Check sheet for the modelled part. Datum: model origin and axes. Units: mm. Give positions to 0.01 mm unless a question says otherwise; leave off trailing zeros. Loops run counter-clockwise (first coordinate to the right, second up) from the corner with the lowest first, then second, coordinate; pieces in that order, holes last. Notation, with made-up numbers: (70, 3.25) -> (128, 3.25) arc R20 ccw to (128, 12.25) -> close; hole circle Ø1 at (76, 86.5). An arc over 180 degrees is marked (long way). Answer as CSV lines item,"result". Start each with the question number.
(1) Gauge pin test, flat ends, axial feed: pin 1 Ø4 at (x, y) = (16, 0.58) entering from -Z; pin 2 Ø5 at (x, y) = (-24, -8) entering from -Z; pin 3 Ø6 at (x, y) = (8, -8) entering from -Z; pin 4 Ø7 at (x, y) = (0, 0.58) entering from -Z. Record the tip position at first contact, or that the pin passes through.
(2) Material ranges on line 1 (Y direction, x = -24, z = 3.15); line 2 (X direction, y = 8, z = 3.2); line 3 (Y direction, x = 9, z = 3.6), recorded low to high. Write a range as from..to.
(3) Section check B-B on x = 65. Enter the section's corners in (y, z), plus the area to 3 significant figures.
(4) Section check C-C on x = -16. Enter the section's corners in (y, z).
(5) Section check A-A on x = 24. Enter the section's corners in (y, z), plus the area to 3 significant figures.
from build123d import *

# Parameters (mm, degrees)
ESQUISSE1_W                                 = 150
ESQUISSE1_H                                 = 30
BOSS_EXTRU_1_DEPTH                          = 4
FRAISAGE_POUR_VIS_T_TE_FRAIS_E_M41_AT_COUNT = 2
FRAISAGE_POUR_VIS_T_TE_FRAIS_E_M41_AT_PITCH = 16
FRAISAGE_POUR_VIS_T_TE_FRAIS_E_M41_2_COUNT  = 2
FRAISAGE_POUR_VIS_T_TE_FRAIS_E_M41_2_PITCH  = 10.908274416
FRAISAGE_POUR_VIS_T_TE_FRAIS_E_M41_3_COUNT  = 2
FRAISAGE_POUR_VIS_T_TE_FRAIS_E_M41_3_PITCH  = 10.908274416
FRAISAGE_POUR_VIS_T_TE_FRAIS_E_M41_4_COUNT  = 2
FRAISAGE_POUR_VIS_T_TE_FRAIS_E_M41_4_PITCH  = 16
FRAISAGE_POUR_VIS_T_TE_FRAIS_E_M41_5_COUNT  = 2
FRAISAGE_POUR_VIS_T_TE_FRAIS_E_M41_5_PITCH  = 22.627416998
FRAISAGE_POUR_VIS_T_TE_FRAIS_E_M41_6_COUNT  = 2
FRAISAGE_POUR_VIS_T_TE_FRAIS_E_M41_6_PITCH  = 25.119523298
FRAISAGE_POUR_VIS_T_TE_FRAIS_E_M41_7_COUNT  = 2
FRAISAGE_POUR_VIS_T_TE_FRAIS_E_M41_7_PITCH  = 16
FRAISAGE_POUR_VIS_T_TE_FRAIS_E_M41_8_COUNT  = 2
FRAISAGE_POUR_VIS_T_TE_FRAIS_E_M41_8_PITCH  = 25.119523298
FRAISAGE_POUR_VIS_T_TE_FRAIS_E_M41_9_COUNT  = 2
FRAISAGE_POUR_VIS_T_TE_FRAIS_E_M41_9_PITCH  = 22.627416998
FRAISAGE_POUR_VIS_T_TE_FRAIS_E_M41_10_COUNT = 2
FRAISAGE_POUR_VIS_T_TE_FRAIS_E_M41_10_PITCH = 32
FRAISAGE_POUR_VIS_T_TE_FRAIS_E_M41_11_COUNT = 2
FRAISAGE_POUR_VIS_T_TE_FRAIS_E_M41_11_PITCH = 40.681573848
FRAISAGE_POUR_VIS_T_TE_FRAIS_E_M41_12_COUNT = 2
FRAISAGE_POUR_VIS_T_TE_FRAIS_E_M41_12_PITCH = 35.77708764
D_GAGEMENT_M61_D                            = 6.6
CONG_1_R                                    = 8
CHANFREIN1_SIZE                             = 0.5


with BuildPart() as part:
    # Esquisse1 → Boss.-Extru.1 (new body)
    with BuildSketch(Plane.XY):
        Rectangle(ESQUISSE1_W, ESQUISSE1_H)
    extrude(amount=BOSS_EXTRU_1_DEPTH)

    # Esquisse3 → Fraisage pour vis à tête fraisée M41 (revolve, cut)
    with BuildSketch(Plane(origin=(8, 8, 0), x_dir=(0, 1, 0), z_dir=(1, 0, 0))):
        Polygon((0, 0), (0, 4), (2.25, 4), (2.25, 2.45), (4.7, 0), align=None)
    fraisage_pour_vis_t_te_frais_e_m41 = revolve(axis=Axis((8, 8, -6.35), (0, 0, 1)), mode=Mode.SUBTRACT)

    # Fraisage pour vis à tête fraisée M41 at: Fraisage pour vis à tête fraisée M41 ×2
    with Locations(*[(0, -i * FRAISAGE_POUR_VIS_T_TE_FRAIS_E_M41_AT_PITCH, 0) for i in range(1, FRAISAGE_POUR_VIS_T_TE_FRAIS_E_M41_AT_COUNT)]):
        add(fraisage_pour_vis_t_te_frais_e_m41, mode=Mode.SUBTRACT)

    # Fraisage pour vis _ t_te frais_e M41 2: Fraisage pour vis à tête fraisée M41 ×2
    with Locations(*[Vector(0.733388224, -0.679810057, 0) * (i * FRAISAGE_POUR_VIS_T_TE_FRAIS_E_M41_2_PITCH) for i in range(1, FRAISAGE_POUR_VIS_T_TE_FRAIS_E_M41_2_COUNT)]):
        add(fraisage_pour_vis_t_te_frais_e_m41, mode=Mode.SUBTRACT)

    # Fraisage pour vis _ t_te frais_e M41 3: Fraisage pour vis à tête fraisée M41 ×2
    with Locations(*[Vector(-0.733388224, -0.679810057, 0) * (i * FRAISAGE_POUR_VIS_T_TE_FRAIS_E_M41_3_PITCH) for i in range(1, FRAISAGE_POUR_VIS_T_TE_FRAIS_E_M41_3_COUNT)]):
        add(fraisage_pour_vis_t_te_frais_e_m41, mode=Mode.SUBTRACT)

    # Fraisage pour vis _ t_te frais_e M41 4: Fraisage pour vis à tête fraisée M41 ×2
    with Locations(*[(-i * FRAISAGE_POUR_VIS_T_TE_FRAIS_E_M41_4_PITCH, 0, 0) for i in range(1, FRAISAGE_POUR_VIS_T_TE_FRAIS_E_M41_4_COUNT)]):
        add(fraisage_pour_vis_t_te_frais_e_m41, mode=Mode.SUBTRACT)

    # Fraisage pour vis _ t_te frais_e M41 5: Fraisage pour vis à tête fraisée M41 ×2
    with Locations(*[Vector(-0.707106781, -0.707106781, 0) * (i * FRAISAGE_POUR_VIS_T_TE_FRAIS_E_M41_5_PITCH) for i in range(1, FRAISAGE_POUR_VIS_T_TE_FRAIS_E_M41_5_COUNT)]):
        add(fraisage_pour_vis_t_te_frais_e_m41, mode=Mode.SUBTRACT)

    # Fraisage pour vis _ t_te frais_e M41 6: Fraisage pour vis à tête fraisée M41 ×2
    with Locations(*[Vector(-0.955432144, -0.295210803, 0) * (i * FRAISAGE_POUR_VIS_T_TE_FRAIS_E_M41_6_PITCH) for i in range(1, FRAISAGE_POUR_VIS_T_TE_FRAIS_E_M41_6_COUNT)]):
        add(fraisage_pour_vis_t_te_frais_e_m41, mode=Mode.SUBTRACT)

    # Fraisage pour vis _ t_te frais_e M41 7: Fraisage pour vis à tête fraisée M41 ×2
    with Locations(*[(i * FRAISAGE_POUR_VIS_T_TE_FRAIS_E_M41_7_PITCH, 0, 0) for i in range(1, FRAISAGE_POUR_VIS_T_TE_FRAIS_E_M41_7_COUNT)]):
        add(fraisage_pour_vis_t_te_frais_e_m41, mode=Mode.SUBTRACT)

    # Fraisage pour vis _ t_te frais_e M41 8: Fraisage pour vis à tête fraisée M41 ×2
    with Locations(*[Vector(0.955432144, -0.295210803, 0) * (i * FRAISAGE_POUR_VIS_T_TE_FRAIS_E_M41_8_PITCH) for i in range(1, FRAISAGE_POUR_VIS_T_TE_FRAIS_E_M41_8_COUNT)]):
        add(fraisage_pour_vis_t_te_frais_e_m41, mode=Mode.SUBTRACT)

    # Fraisage pour vis _ t_te frais_e M41 9: Fraisage pour vis à tête fraisée M41 ×2
    with Locations(*[Vector(0.707106781, -0.707106781, 0) * (i * FRAISAGE_POUR_VIS_T_TE_FRAIS_E_M41_9_PITCH) for i in range(1, FRAISAGE_POUR_VIS_T_TE_FRAIS_E_M41_9_COUNT)]):
        add(fraisage_pour_vis_t_te_frais_e_m41, mode=Mode.SUBTRACT)

    # Fraisage pour vis _ t_te frais_e M41 10: Fraisage pour vis à tête fraisée M41 ×2
    with Locations(*[(-i * FRAISAGE_POUR_VIS_T_TE_FRAIS_E_M41_10_PITCH, 0, 0) for i in range(1, FRAISAGE_POUR_VIS_T_TE_FRAIS_E_M41_10_COUNT)]):
        add(fraisage_pour_vis_t_te_frais_e_m41, mode=Mode.SUBTRACT)

    # Fraisage pour vis _ t_te frais_e M41 11: Fraisage pour vis à tête fraisée M41 ×2
    with Locations(*[Vector(-0.983246129, -0.182282885, 0) * (i * FRAISAGE_POUR_VIS_T_TE_FRAIS_E_M41_11_PITCH) for i in range(1, FRAISAGE_POUR_VIS_T_TE_FRAIS_E_M41_11_COUNT)]):
        add(fraisage_pour_vis_t_te_frais_e_m41, mode=Mode.SUBTRACT)

    # Fraisage pour vis _ t_te frais_e M41 12: Fraisage pour vis à tête fraisée M41 ×2
    with Locations(*[Vector(-0.894427191, -0.447213595, 0) * (i * FRAISAGE_POUR_VIS_T_TE_FRAIS_E_M41_12_PITCH) for i in range(1, FRAISAGE_POUR_VIS_T_TE_FRAIS_E_M41_12_COUNT)]):
        add(fraisage_pour_vis_t_te_frais_e_m41, mode=Mode.SUBTRACT)

    # Dégagement M61 (through all)
    with Locations(Plane(origin=(0, 0, 0), x_dir=(-1, 0, 0), z_dir=(0, 0, -1))):
        with Locations((-65, 0), (65, 0)):
            Hole(D_GAGEMENT_M61_D / 2)

    # Congé1
    cong_1_edges = [part.edges().sort_by_distance(p)[0] for p in [
        (-75, 15, 2),
        (75, 15, 2),
        (75, -15, 2),
        (-75, -15, 2),
    ]]
    fillet(cong_1_edges, radius=CONG_1_R)

    # Chanfrein1
    chanfrein1_edges = [part.edges().sort_by_distance(p)[0] for p in [
        (0, 15, 0),
        (0, 15, 4),
        (-75, 0, 0),
        (75, 0, 0),
        (0, -15, 0),
        (-72.656854249, 12.656854249, 0),
        (-72.656854249, -12.656854249, 0),
        (72.656854249, -12.656854249, 0),
        (72.656854249, 12.656854249, 0),
        (75, 0, 4),
        (-75, 0, 4),
        (0, -15, 4),
        (-72.656854249, 12.656854249, 4),
        (-72.656854249, -12.656854249, 4),
        (72.656854249, -12.656854249, 4),
        (72.656854249, 12.656854249, 4),
    ]]
    chamfer(chanfrein1_edges, length=CHANFREIN1_SIZE)


solid = part.part
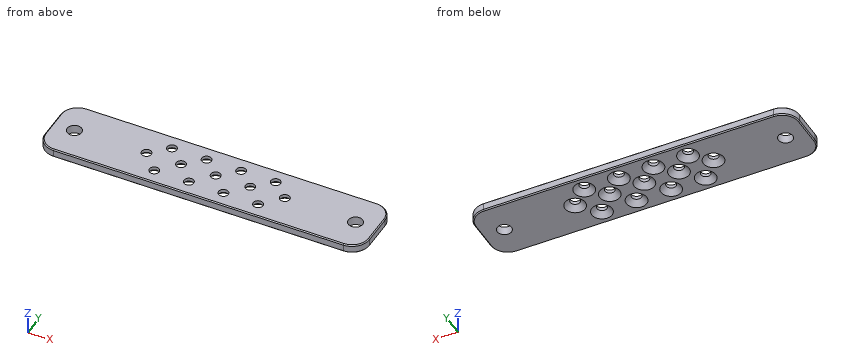
Working result:
1,pin 1,"passes through"
1,pin 2,"stops at z = 2.2"
1,pin 3,"stops at z = 1.7"
1,pin 4,"stops at z = 1.2"
2,line 1,"y = -15..-10.25, -5.75..5.75, 10.25..15"
2,line 2,"x = -74.94..-26.25, -21.75..-10.25, -5.75..5.75, 10.25..21.75, 26.25..74.94"
2,line 3,"y = -14.9..-10.02, -5.98..5.98, 10.02..14.9"
3,outline,"(-15, 0.5) -> (-14.5, 0) -> (-3.3, 0) -> (-3.3, 4) -> (-14.5, 4) -> (-15, 3.5) -> close; (3.3, 0) -> (14.5, 0) -> (15, 0.5) -> (15, 3.5) -> (14.5, 4) -> (3.3, 4) -> close"
3,area,"93.1 mm^2"
4,outline,"(-15, 0.5) -> (-14.5, 0) -> (-4.12, 0) -> (-1.67, 2.45) -> (-1.67, 4) -> (-14.5, 4) -> (-15, 3.5) -> close; (2.83, 2.45) -> (5.28, 0) -> (14.5, 0) -> (15, 0.5) -> (15, 3.5) -> (14.5, 4) -> (2.83, 4) -> close"
5,outline,"(-15, 0.5) -> (-14.5, 0) -> (-12.7, 0) -> (-10.25, 2.45) -> (-10.25, 4) -> (-14.5, 4) -> (-15, 3.5) -> close; (-5.75, 2.45) -> (-3.3, 0) -> (3.3, 0) -> (5.75, 2.45) -> (5.75, 4) -> (-5.75, 4) -> close; (10.25, 2.45) -> (12.7, 0) -> (14.5, 0) -> (15, 0.5) -> (15, 3.5) -> (14.5, 4) -> (10.25, 4) -> close"
5,area,"71.5 mm^2"
